```python
from build123d import *

# Parameters (mm, degrees)
SKETCH1_R           = 1.5875
BOSS_EXTRUDE1_DEPTH = 9.525
SKETCH3_W           = 15
SKETCH3_H           = 3.175
SKETCH3_W_2         = 5
BOSS_EXTRUDE2_DEPTH = 12.7


with BuildPart() as part:
    # Sketch1 → Boss-Extrude1 (new body)
    with BuildSketch(Plane(origin=(0, 0, 0), x_dir=(0, 0, -1), z_dir=(1, 0, 0))):
        Polygon((0, 1.5875), (0, -1.5875), (-25.4, -1.5875), (-25.4, -4.7625), (-38.1, -4.7625), (-38.1, -1.5875), (-76.2, -1.5875), (-76.2, 1.5875), align=None)
        with Locations((-31.75, -1.5875)):
            Circle(SKETCH1_R, mode=Mode.SUBTRACT)
    extrude(amount=BOSS_EXTRUDE1_DEPTH)

    # Sketch3 → Boss-Extrude2 (add, symmetric)
    with BuildSketch(Plane(origin=(4.7625, 0, 0), x_dir=(0, 0, -1), z_dir=(1, 0, 0))):
        with Locations((-68.7, 0)):
            Rectangle(SKETCH3_W, SKETCH3_H)
        with Locations((-78.7, 0)):
            Rectangle(SKETCH3_W_2, SKETCH3_H)
    extrude(amount=BOSS_EXTRUDE2_DEPTH, both=True)


solid = part.part
```
The listing builds one solid part. Answer for the finished solid, in the listing's coordinates (mm). A direction names the side the tool comes from. Coordinates: 2 decimals unless noted, no trailing zeros. Write each loop counter-clockwise with the first axis right and the second up, starting at its lowest first coordinate (ties: lowest second). Pieces come first, ordered by that corner, then holes. Notation, with made-up numbers: (74.25, 12) - (87.25, 12) arc R27 cw to (87.25, 30) - close; hole circle Ø1 at (-2, 75.5). An arc over 180 degrees is marked (long way). One line per item, written item: value.
1) Find section A-A (z = 31.75). Give the vertices of the cut face in (x, y) (1 decimal), and give its area (3 significant figures).
Geometry check:
outline: (0, -4.8) - (9.5, -4.8) - (9.5, -3.2) - (0, -3.2) - close; (0, 0) - (9.5, 0) - (9.5, 1.6) - (0, 1.6) - close
area: 30.2 mm2
2) Each of these flat-tipped pins is pushed along its axis until it touches: pin 1 Ø3 at (x, z) = (4, 14.5) entering from -Y; pin 2 Ø1 at (x, y) = (6.5, -3) entering from -Z; pin 3 Ø1.9 at (y, z) = (-3, 33.5) entering from -X; pin 4 Ø3 at (x, y) = (7, -2.5) entering from +Z. Where does it stop, or does it pass through?
Geometry check:
pin 1: stops at y = -1.59
pin 2: stops at z = 25.4
pin 3: stops at x = 0
pin 4: stops at z = 81.2
3) Find section D-D (z = 55.5). Give the vertices of the cut face in (x, y) (1 decimal), and give its area (3 significant figures).
Geometry check:
outline: (0, -1.6) - (9.5, -1.6) - (9.5, 1.6) - (0, 1.6) - close
area: 30.2 mm2
4) For a pull along Y with two mould halves and no side action, classify faces 1 (the flat face through (-7.937, 0, 71)), 2 (the cylindrical face through (4.696, -1.111, 30.236)), 3 (the flat face through (5, 1.588, 49)) as pulls with the +Y half, pulls with the -Y half, needs draft (parallel to the pull), parting line crosses it, or undercut.
Geometry check:
face 1: needs draft
face 2: undercut
face 3: pulls with the +Y half
5) Find section C-C (x = -4.5). Give the vertices of the cut face in (y, z).
Geometry check:
outline: (-1.59, 61.2) - (1.59, 61.2) - (1.59, 81.2) - (-1.59, 81.2) - close
6) Consider line 1 along Y through (x, z) = (5, 31.75) (1 decimal); line 2 along Z through (x, y) = (10.5, -1.25); line 3 along X through (y, z) = (1.5, 30.5) (3 decimals). Determine where each line is inside the solid, lowest interval first. Write a range as from..to.
Geometry check:
line 1: y = -4.8..-3.2, 0..1.6
line 2: z = 61.2..81.2
line 3: x = 0..9.525
7) A tool of negligible diameter and unlimited length cuts with its end or side. For faces 4 (the flat face through (5, -1.588, 65)), 5 (the flat face through (5, -1.588, 13)), 6 (the flat face through (0, -1, 30)), 7 (the flat face through (9.525, -1, 30)), from which of +Z, -Z, +X, -X, +Y, -Y can it reach the whole face along a straight path? Write none if from no direction.
Geometry check:
face 4: +Z, +X, -X, -Y
face 5: -Z, +X, -X, -Y
face 6: -Z, -X, +Y, -Y
face 7: -Z, +X, +Y, -Y
